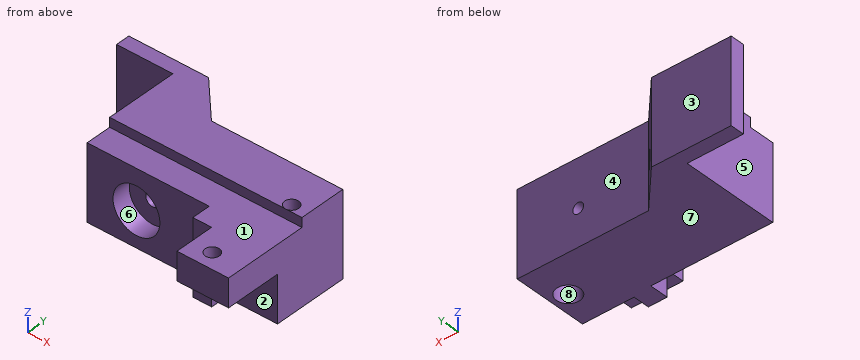
```python
from build123d import *

# Parameters (mm, degrees)
SKETCH1_W           = 41
SKETCH1_H           = 28
BOSS_EXTRUDE1_DEPTH = 18
CUT_EXTRUDE1_DEPTH  = 18
BOSS_EXTRUDE2_DEPTH = 18
SKETCH4_W           = 41
SKETCH4_H           = 18
CUT_EXTRUDE2_DEPTH  = 2
SKETCH5_R           = 1.5
CUT_EXTRUDE9_DEPTH  = 11
SKETCH6_R           = 1.5
CUT_EXTRUDE10_DEPTH = 43.64387412
SKETCH7_R           = 2.5
CUT_EXTRUDE11_DEPTH = 7
SKETCH8_W           = 11
SKETCH8_H           = 12
CUT_EXTRUDE12_DEPTH = 10
SKETCH9_R           = 5
CUT_EXTRUDE13_DEPTH = 4
SKETCH10_R          = 1.5
CUT_EXTRUDE14_DEPTH = 43.1930089
SKETCH11_R          = 1.15
CUT_EXTRUDE15_DEPTH = 47.521500406


with BuildPart() as part:
    # Sketch1 → Boss-Extrude1 (new body)
    with BuildSketch(Plane.XY):
        Rectangle(SKETCH1_W, SKETCH1_H)
    extrude(amount=BOSS_EXTRUDE1_DEPTH)

    # Sketch2 → Cut-Extrude1 (cut)
    with BuildSketch(Plane.XY.offset(18)):
        Polygon((9.5, -14), (9.5, -5.5), (5.5, -5.5), (5.5, -1.5), (-20.5, -1.5), (-20.5, -14), align=None)
    extrude(amount=-CUT_EXTRUDE1_DEPTH, mode=Mode.SUBTRACT)

    # Sketch3 → Boss-Extrude2 (add)
    with BuildSketch(Plane.XY.offset(18)):
        Polygon((-20.5, 22.5), (-32.5, 22.5), (-32.5, 19.5), (-20.5, 19.5), (-20.5, 14), (-7.5, 14), (-15.5, 22.5), align=None)
    extrude(amount=-BOSS_EXTRUDE2_DEPTH)

    # Sketch4 → Cut-Extrude2 (cut)
    with BuildSketch(Plane.XY.offset(18)):
        with Locations((0, -5)):
            Rectangle(SKETCH4_W, SKETCH4_H)
    extrude(amount=-CUT_EXTRUDE2_DEPTH, mode=Mode.SUBTRACT)

    # Sketch5 → Cut-Extrude9 (cut)
    with BuildSketch(Plane.XY.offset(18)):
        with Locations((17, 5.501)):
            Circle(SKETCH5_R)
    extrude(amount=-CUT_EXTRUDE9_DEPTH, mode=Mode.SUBTRACT)

    # Sketch6 → Cut-Extrude10 (cut, through all)
    with BuildSketch(Plane.XY.offset(16)):
        with Locations((14, -10.5)):
            Circle(SKETCH6_R)
    extrude(amount=-CUT_EXTRUDE10_DEPTH, mode=Mode.SUBTRACT)

    # Sketch7 → Cut-Extrude11 (cut)
    with BuildSketch(Plane(origin=(0, 0, 0), x_dir=(-1, 0, 0), z_dir=(0, 0, -1))):
        with Locations((-17, 5.501)):
            Circle(SKETCH7_R)
    extrude(amount=-CUT_EXTRUDE11_DEPTH, mode=Mode.SUBTRACT)

    # Sketch8 → Cut-Extrude12 (cut)
    with BuildSketch(Plane(origin=(0, 0, 0), x_dir=(-1, 0, 0), z_dir=(0, 0, -1))):
        with Locations((-15, -8)):
            Rectangle(SKETCH8_W, SKETCH8_H)
    extrude(amount=-CUT_EXTRUDE12_DEPTH, mode=Mode.SUBTRACT)

    # Sketch9 → Cut-Extrude13 (cut)
    with BuildSketch(Plane.XZ.offset(1.5)):
        with Locations((-10, 7.5)):
            Circle(SKETCH9_R)
    extrude(amount=-CUT_EXTRUDE13_DEPTH, mode=Mode.SUBTRACT)

    # Sketch10 → Cut-Extrude14 (cut, through all)
    with BuildSketch(Plane.XZ.offset(-2.5)):
        with Locations((-10, 7.5)):
            Circle(SKETCH10_R)
    extrude(amount=-CUT_EXTRUDE14_DEPTH, mode=Mode.SUBTRACT)

    # Sketch11 → Cut-Extrude15 (cut, through all)
    with BuildSketch(Plane.XZ.offset(5.5)):
        with Locations((7.5, 7.85)):
            Circle(SKETCH11_R)
    extrude(amount=-CUT_EXTRUDE15_DEPTH, mode=Mode.SUBTRACT)


solid = part.part
```
CAD build for the part. Positions are in the model's coordinates, mm. Face numbers are marked on the shaded views. A direction names the side the tool comes from. Coordinates: 2 decimals unless noted, no trailing zeros. Order: outer loops, then holes, each group sorted by start corner. A loop starts at its lowest first (then second) coordinate and runs counter-clockwise, first axis right, second up. Notation, with made-up numbers: M 73.5,72.25 L 90.5,72.25 A4 ccw 90.5,78.25 Z; hole C 38.5,75 d2. An arc over 180 degrees is marked long. Write each question's results on one line, items separated by ' | '. Start each with the question number.
Q1. Pull direction Z, two halves, no side cores. Call the marked faces 6, 7 and 8: +Z half, -Z half, draft (parallel to the pull), parting line (faces both ways), or undercut.
Q2. Drill centre lines: probe 1 along Z at (x, y) = (-10, 8); probe 2 along Y at (x, z) = (17, 11.75); probe 3 along Z at (x, y) = (7.5, -0.5). Where is each one in solid material? Low to high. Write a range as from..to.
Q3. Which spindle directions (+Z, -Z, +X, -X, +Y, -Y) get a long thin tool onto all of the face, cutting with end or side? Do the marked faces 1, 2, 3, 4 and 5. Say none if no direction does.
Q4. Cut at D-D (x = 1.5). List the corners of the cut face in (y, z).
Q5. Flat gauge pins, fed straight in: P1, Ø1, axis at x = 6, z = 14, coming from the +Y side; P2, Ø3, axis at x = -8.5, z = 6.5, coming from the +Y side; P3, Ø2.5, axis at x = 17, y = 5.501, coming from the +Z side; P4, Ø1, axis at y = -4.5, z = 3, coming from the +X side. Where does each tip first touch, or does it go through?
Q6. Cut at A-A (x = 7.5). List the corners of the cut face in (y, z), then the cut area to 3 significant figures.
Q7. Cut at B-B (y = 13). List the corners of the cut face in (x, z), then the cut area to 3 significant figures.
Q8. Cut at C-C (z = 4). List the corners of the cut face in (x, y).
Found:
1) face 6: undercut | face 7: -Z half | face 8: draft
2) probe 1: 0..6, 9..18 | probe 2: -14..4, 7..14 | probe 3: 0..6.7, 9..16
3) face 1: +Z, +X, -X, -Y | face 2: -Z, +X, -Y | face 3: +Z, -Z, +X, -X, +Y | face 4: +Z, -Z, +X, +Y | face 5: +Z, -Z, -X, -Y
4) outline: M -1.5,0 L 14,0 L 14,18 L 4,18 L 4,16 L -1.5,16 Z
5) P1: y = 14 | P2: y = 16.57 | P3: through | P4: x = 9.5
6) outline: M -5.5,0 L 14,0 L 14,6.7 L -5.5,6.7 Z; M -5.5,9 L 14,9 L 14,18 L 4,18 L 4,16 L -5.5,16 Z | area: 287 mm²
7) outline: M -20.5,0 L 20.5,0 L 20.5,18 L -20.5,18 Z; hole C -10,7.5 d3; hole C 7.5,7.85 d2.3 | area: 727 mm²
8) outline: M -32.5,19.5 L -20.5,19.5 L -20.5,-1.5 L -13.57,-1.5 L -13.57,2.5 L -6.43,2.5 L -6.43,-1.5 L 5.5,-1.5 L 5.5,-5.5 L 9.5,-5.5 L 9.5,-2 L 20.5,-2 L 20.5,14 L -7.5,14 L -15.5,22.5 L -32.5,22.5 Z; hole C 17,5.5 d5
